The drawing under review shows one solid part. Ordinate dimensions are in mm from its lowest x, y, z. Coordinates: 2 decimals unless noted, no trailing zeros. Write each loop counter-clockwise with the first axis right and the second up, starting at its lowest first coordinate (ties: lowest second). Pieces come first, ordered by that corner, then holes.
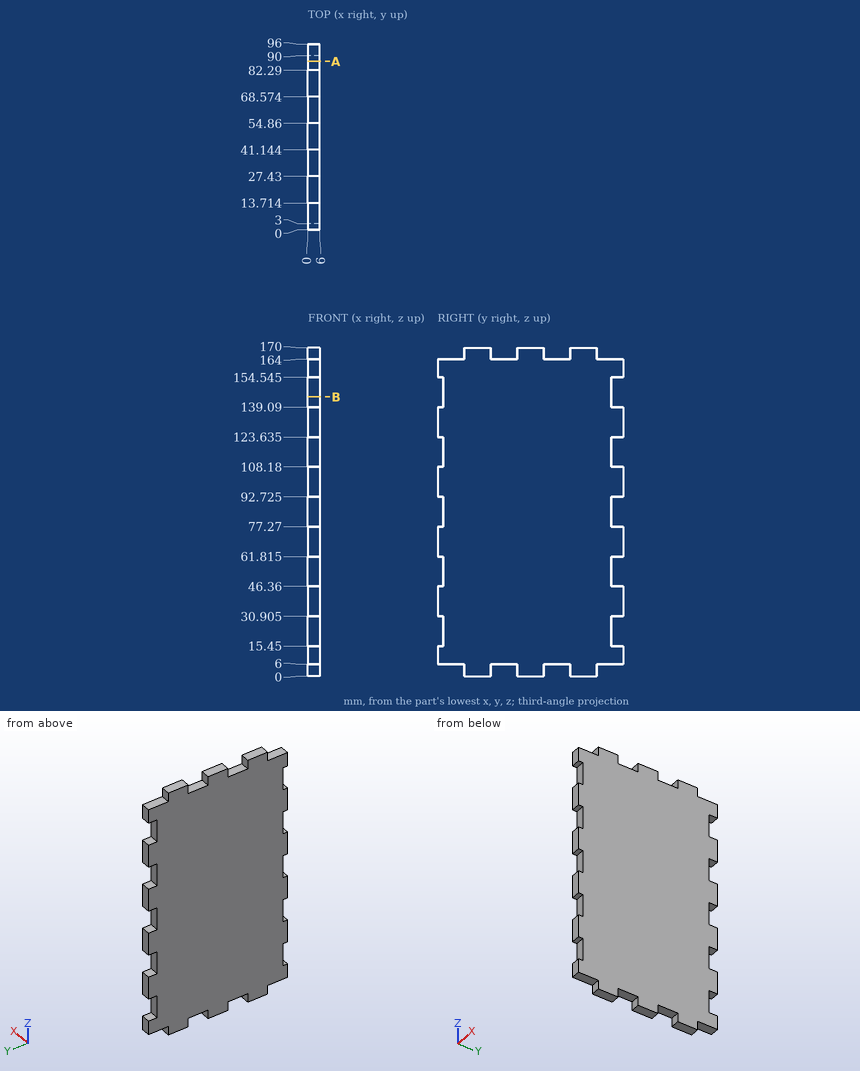
Q1. For probe 1 along Z at (x, y) = (3.65, 66); probe 2 along Y at (x, z) = (5.65, 121), list the stretches that pass through material, from the lowest coordinate up.
Ans:
probe 1: z = 6 to 164
probe 2: y = 3 to 90
Q2. Clearance check with flat-ended pins moving along their axes: pin 1 Ø3 at (x, y) = (4.5, 90) entering from -Z; pin 2 Ø1.8 at (x, z) = (3, 166.5) entering from -Y; pin 3 Ø1.5 at (x, y) = (3, 1.5) entering from +Z. State where each tip first meets the part, or that it passes through.
Ans:
pin 1: stops at z = 6
pin 2: stops at y = 13.71
pin 3: stops at z = 164
Q3. Add section B-B (z = 144.5). State the section outline as (x, y) points.
Ans:
outline: (0, 3) - (6, 3) - (6, 90) - (0, 90) - close
Q4. Add section A-A (y = 87). State the section outline as (x, z) points, then the cut area to 3 significant figures.
Ans:
outline: (0, 6) - (6, 6) - (6, 164) - (0, 164) - close
area: 948 mm2
